```python
from build123d import *

# Parameters (mm, degrees)
BOSS_EXTRUDE1_DEPTH = 20
CUT_EXTRUDE19_DEPTH = 45
CUT_EXTRUDE23_DEPTH = 444
SKETCH10_W          = 25.4
SKETCH10_H          = 2
CUT_EXTRUDE25_DEPTH = 45
CUT_EXTRUDE26_DEPTH = 444
SKETCH16_R          = 3.25
SKETCH16_R_2        = 3.15
CUT_EXTRUDE28_DEPTH = 45
SKETCH18_R          = 3.15
CUT_EXTRUDE30_DEPTH = 20
CUT_EXTRUDE31_DEPTH = 6.15


with BuildPart() as part:
    # Sketch1 → Boss-Extrude1 (new body)
    with BuildSketch(Plane(origin=(0, 0, 0), x_dir=(1, 0, 0), z_dir=(0, 1, 0))):
        Polygon((-22.5, -50), (22.5, -50), (22.5, 10), (17.5, 10), (17.5, -10), (12.5, -10), (12.5, 10), (7.5, 10), (7.5, -10), (2.5, -10), (-2.5, -10), (-7.5, -10), (-7.5, 10), (-12.5, 10), (-12.5, -10), (-17.5, -10), (-17.5, 10), (-22.5, 10), align=None)
    extrude(amount=BOSS_EXTRUDE1_DEPTH)

    # Sketch6 → Cut-Extrude19 (cut)
    with BuildSketch(Plane(origin=(22.5, 0, 0), x_dir=(0, 0, -1), z_dir=(1, 0, 0))):
        with BuildLine():
            ThreePointArc((10, 8.5), (7.51040764, 2.48959236), (1.5, 0))
            Line((1.5, 0), (10, 0))
            Line((10, 0), (10, 8.5))
        make_face()
        with BuildLine():
            ThreePointArc((1.5, 17), (7.51040764, 14.51040764), (10, 8.5))
            Line((10, 8.5), (10, 20))
            Line((10, 20), (-10, 20))
            Line((-10, 20), (-10, 17))
            Line((-10, 17), (1.5, 17))
        make_face()
    extrude(amount=-CUT_EXTRUDE19_DEPTH, mode=Mode.SUBTRACT)

    # Sketch2 → Cut-Extrude23 (cut)
    with BuildSketch(Plane.XY.offset(50)):
        with BuildLine():
            Line((-22.5, 20), (22.5, 20))
            Line((22.5, 20), (22.5, 16))
            ThreePointArc((22.5, 16), (20.832845478, 17.631987193), (18.5, 17.607120136))
            ThreePointArc((18.5, 17.607120136), (0, 13.071891388), (-18.5, 17.607120136))
            ThreePointArc((-18.5, 17.607120136), (-20.832845478, 17.631987193), (-22.5, 16))
            Line((-22.5, 16), (-22.5, 20))
        make_face()
    extrude(amount=-CUT_EXTRUDE23_DEPTH, mode=Mode.SUBTRACT)

    # Sketch10 → Cut-Extrude25 (cut)
    with BuildSketch(Plane.ZY.offset(22.5)):
        Polygon((37.7, 10), (37.7, 8), (12.3, 8), (12.3, 10), (25, 10), align=None)
        with Locations((-25, 9)):
            Rectangle(SKETCH10_W, SKETCH10_H)
        Polygon((-303.835718962, 8), (-292.208543952, 8), (-279.508543952, 8), (-279.508543952, 10), (-292.208543952, 10), (-303.835718962, 10), align=None)
        Polygon((-329.508543952, 10), (-329.508543952, 8), (-354.908543952, 8), (-354.908543952, 10), (-342.208543952, 10), align=None)
        Polygon((-229.508543952, 8), (-254.908543952, 8), (-254.908543952, 10), (-242.208543952, 10), (-229.508543952, 10), align=None)
    extrude(amount=-CUT_EXTRUDE25_DEPTH, mode=Mode.SUBTRACT)

    # Sketch12 → Cut-Extrude26 (cut)
    with BuildSketch(Plane.XY.offset(50)):
        Polygon((-1, 3.35), (-1, 6.55), (0, 6.55), (1, 6.55), (1, 3.35), align=None)
    extrude(amount=-CUT_EXTRUDE26_DEPTH, mode=Mode.SUBTRACT)

    # Sketch16 → Cut-Extrude28 (cut)
    with BuildSketch(Plane.ZY.offset(22.5)):
        with Locations((-1.25, 8.5)):
            Circle(SKETCH16_R)
        with Locations((-386.058543952, 2.588831384)):
            Circle(SKETCH16_R_2)
    extrude(amount=-CUT_EXTRUDE28_DEPTH, mode=Mode.SUBTRACT)

    # Sketch18 → Cut-Extrude30 (cut)
    with BuildSketch(Plane.XZ):
        with Locations((-3.5, 43.85)):
            Circle(SKETCH18_R)
    extrude(amount=-CUT_EXTRUDE30_DEPTH, mode=Mode.SUBTRACT)

    # Sketch24 → Cut-Extrude31 (cut)
    with BuildSketch(Plane.XY.offset(50)):
        Polygon((-1, 6.55), (-11, 6.55), (-22.5, 6.55), (-22.5, 3.35), (-11, 3.35), (-1, 3.35), (1, 3.35), (11, 3.35), (22.5, 3.35), (22.5, 6.55), (11, 6.55), (1, 6.55), align=None)
    extrude(amount=-CUT_EXTRUDE31_DEPTH, mode=Mode.SUBTRACT)


solid = part.part
```
Here's how the part is built. I have some questions about the finished solid (model axes, mm). A direction names the side the tool comes from. Round coordinates to 2 decimals unless told otherwise and drop trailing zeros. Loops run counter-clockwise (first coordinate to the right, second up) from the corner with the lowest first, then second, coordinate; pieces in that order, holes last.
1. Suppose I cut it at C-C, the plane z = 8.5. Please give me the cut outline in (x, y).
Answers:
outline: (-22.5, 0) - (-17.5, 0) - (-17.5, 17) - (-21.81, 17) arc R3.05 ccw to (-22.5, 16) - close; (-12.5, 0) - (-7.5, 0) - (-7.5, 13.78) arc R40 cw to (-12.5, 15.08) - close; (7.5, 0) - (12.5, 0) - (12.5, 15.08) arc R40 cw to (7.5, 13.78) - close; (17.5, 0) - (22.5, 0) - (22.5, 16) arc R3.05 ccw to (21.81, 17) - (17.5, 17) - close
2. Suppose I cut it at A-A, the plane z = 25. Please give me the cut outline in (x, y).
Answers:
outline: (-22.5, 0) - (22.5, 0) - (22.5, 8) - (-22.5, 8) - close; (-22.5, 10) - (22.5, 10) - (22.5, 16) arc R3.05 ccw to (18.5, 17.61) arc R40 cw to (-18.5, 17.61) arc R3.05 ccw to (-22.5, 16) - close; hole (-1, 3.35) - (1, 3.35) - (1, 6.55) - (-1, 6.55) - close
3. Will these pins go through, and if not, where does the flat tip stop? pin 1 (5 mm diameter, centred on x = -2, z = 38.5, fed in from +Y); pin 2 (2 mm diameter, centred on x = 5, y = 6, fed in from -Z); pin 3 (8 mm diameter, centred on x = -7, z = 27.5, fed in from +Y); pin 4 (4 mm diameter, centred on x = -3.5, z = 43.85, fed in from +Y).
Answers:
pin 1: stops at y = 13.33
pin 2: stops at z = 10
pin 3: stops at y = 14.61
pin 4: passes through
4. Suppose I cut it at D-D, the plane z = -3. Give the number of separate pieces and of enclosed holes in the cut face, and give its area (3 significant figures).
Answers:
separate pieces: 8
enclosed holes: 0
area: 200 mm2
5. If I drill on probe 1 along X at (y, z) = (4.5, 21); probe 2 along Y at (x, z) = (20.1, -1.25); probe 3 along X at (y, z) = (3, 43.85), over which ranges is the centre line in solid material (lowest first)?
Answers:
probe 1: x = -22.5 to -1, 1 to 22.5
probe 2: y = 0 to 5.25, 11.75 to 17
probe 3: x = -22.5 to -6.65, -0.35 to 22.5
6. Thinking about a two-plate mould opening in Y: for faces 5 (the face through (20, 17, 4)), 6 (the face through (22.5, 6, 20)), 7 (the face through (0, 6.55, 43)), which applies, released by +Y, released by -Y, zero draft, split by the parting line, or undercut?
Answers:
face 5: released by +Y
face 6: zero draft
face 7: undercut
7. Suppose I cut it at B-B, the plane x = -3.5. Please give me the cut outline in (y, z).
Answers:
outline: (0, 10) - (13.23, 10) - (13.23, 40.7) - (0, 40.7) - close; (0, 47) - (3.35, 47) - (3.35, 50) - (0, 50) - close; (6.55, 47) - (13.23, 47) - (13.23, 50) - (6.55, 50) - close; hole (8, 12.3) - (10, 12.3) - (10, 37.7) - (8, 37.7) - close
8. For faces 1 (the face through (1, 5, 27)), 2 (the face through (0, 8, 25)), 3 (the face through (-17.5, 8.4, 2.4)), 4 (the face through (-15, 5, 43.85)), which set-ups out of +Z, -Z, +X, -X, +Y, -Y let a thin tool reach every point of the face, with its end or its side?
Answers:
face 1: +Z, -Z
face 2: +X, -X
face 3: -Z, +Y, -Y
face 4: +Z, +X, -X
